Here's how the part is built. I have some questions about the finished solid (model axes, mm). A direction names the side the tool comes from. Give positions to 0.01 mm unless a question says otherwise; leave off trailing zeros. Order: outer loops, then holes, each group sorted by start corner. A loop starts at its lowest first (then second) coordinate and runs counter-clockwise, first axis right, second up.
from build123d import *

# Parameters (mm, degrees)
SKETCH_1_W      = 16.5
SKETCH_1_H      = 15.4
SKETCH_1_R      = 0.5
EXTRUDE_1_DEPTH = 7.5
SKETCH_2_W      = 12
SKETCH_2_H      = 2.7
EXTRUDE_2_DEPTH = 2
SKETCH_3_W      = 12
SKETCH_3_H      = 0.5
EXTRUDE_3_DEPTH = 6
SKETCH_4_R      = 2
EXTRUDE_4_DEPTH = 11.45


with BuildPart() as part:
    # 草图1 → 凸台-拉伸1 (new body)
    with BuildSketch(Plane(origin=(0, 0, 0), x_dir=(1, 0, 0), z_dir=(0, 1, 0))):
        with Locations((0.25, 0.05)):
            Rectangle(SKETCH_1_W, SKETCH_1_H)
        with Locations(Location((0, 0, 0), (0, 0, 270))):
            Circle(SKETCH_1_R, mode=Mode.SUBTRACT)
    extrude(amount=EXTRUDE_1_DEPTH)

    # 草图2 → 凸台-拉伸2 (add)
    with BuildSketch(Plane.XZ):
        with Locations((2.5, 9)):
            Rectangle(SKETCH_2_W, SKETCH_2_H)
    extrude(amount=-EXTRUDE_2_DEPTH)

    # 草图3 → 凸台-拉伸3 (add)
    with BuildSketch(Plane(origin=(0, 2, 0), x_dir=(1, 0, 0), z_dir=(0, 1, 0))):
        with Locations((2.5, -10.1)):
            Rectangle(SKETCH_3_W, SKETCH_3_H)
    extrude(amount=-EXTRUDE_3_DEPTH)

    # 草图4 → 凸台-拉伸4 (add)
    with BuildSketch(Plane(origin=(0, 7.5, 0), x_dir=(1, 0, 0), z_dir=(0, 1, 0))):
        with Locations(Location((0, 0, 0), (0, 0, 270))):
            Circle(SKETCH_4_R)
    extrude(amount=EXTRUDE_4_DEPTH)

    # 草图5 → 旋转1 (revolve)
    with BuildSketch(Plane.XY):
        with BuildLine():
            Line((0, 9), (5.137119816, 9))
            ThreePointArc((5.137119816, 9), (5.780256002, 7.508925279), (6, 5.9))
            Line((6, 5.9), (0, 5.9))
            Line((0, 5.9), (0, 9))
        make_face()
    revolve(axis=Axis((0, 0, 0), (0, 1, 0)))


solid = part.part
Q1. If we section it at B-B on z = 0: List the corners of the cut face in (x, y) for me, plus the area to 3 significant figures.
Filled sheet:
outline: (-8, 0) - (-0.5, 0) - (-0.5, 5.9) - (0.5, 5.9) - (0.5, 0) - (8.5, 0) - (8.5, 7.5) - (5.78, 7.5) arc R6 ccw to (5.14, 9) - (2, 9) - (2, 18.95) - (-2, 18.95) - (-2, 9) - (-5.14, 9) arc R6 ccw to (-5.78, 7.5) - (-8, 7.5) - close
area: 174 mm2
Q2. If we section it at D-D on y = -2: List the corners of the cut face in (x, z) for me.
Filled sheet:
outline: (-3.5, 9.85) - (8.5, 9.85) - (8.5, 10.35) - (-3.5, 10.35) - close
Q3. Thinking about a two-plate mould opening in X: for faces 6 (the face through (0, 4, -7.75)), 7 (the face through (0, 5.9, 0)), 8 (the face through (-3.5, 0.4, 9.3)), which applies, released by +X, released by -X, zero draft, split by the parting line, or undercut?
Filled sheet:
face 6: zero draft
face 7: undercut
face 8: released by -X
Q4. For faces 1 (the face through (2, -2, 9.85)), 2 (the face through (2, -1, 10.35)), 3 (the face through (-2.2, 9, -0.1)), 4 (the face through (-0.488, 2.909, -0.108)), 5 (the face through (2, 2, 9)), which set-ups out of +Z, -Z, +X, -X, +Y, -Y let a thin tool reach every point of the face, with its end or its side?
Filled sheet:
face 1: -Z, +X, -X, -Y
face 2: +Z, +X, -X, +Y, -Y
face 3: +Y
face 4: -Y
face 5: +Z, +X, -X, +Y
Q5. I need wall thicknesses on L1, parallel to Z at x = 0, y = 1.35; L2, parallel to Z at x = 0, y = 4.05; L3, parallel to X at y = 2.7, z = 0. Which ranges of each line are inside material? Lowest first, please.
Filled sheet:
L1: z = -7.75 to -0.5, 0.5 to 10.35
L2: z = -7.75 to -0.5, 0.5 to 7.65
L3: x = -8 to -0.5, 0.5 to 8.5
Q6. If we section it at A-A on y = 3: List the corners of the cut face in (x, z) for me.
Filled sheet:
outline: (-8, -7.75) - (8.5, -7.75) - (8.5, 7.65) - (-8, 7.65) - close; hole circle Ø1 at (0, 0)
Q7. I'm going to push flat-ended pins straight in: P1, Ø4, axis at x = -0.5, y = 13, coming from the -Z side; P2, Ø8, axis at y = 15, z = 1.5, coming from the +X side; P3, Ø2, axis at x = 5, z = 8.5, coming from the +Y side; P4, Ø8, axis at y = 16, z = 6.5, coming from the +X side. Where does each tip first touch, or does it pass through?
Filled sheet:
P1: stops at z = -2
P2: stops at x = 2
P3: stops at y = 7.5
P4: passes through
Q8. If we section it at C-C on x = 0: List the corners of the cut face in (y, z) for me.
Filled sheet:
outline: (-4, 9.85) - (0, 9.85) - (0, 0.5) - (5.9, 0.5) - (5.9, -0.5) - (0, -0.5) - (0, -7.75) - (7.5, -7.75) - (7.5, -5.78) arc R6 ccw to (9, -5.14) - (9, -2) - (18.95, -2) - (18.95, 2) - (9, 2) - (9, 5.14) arc R6 ccw to (7.5, 5.78) - (7.5, 7.65) - (2, 7.65) - (2, 10.35) - (-4, 10.35) - close
